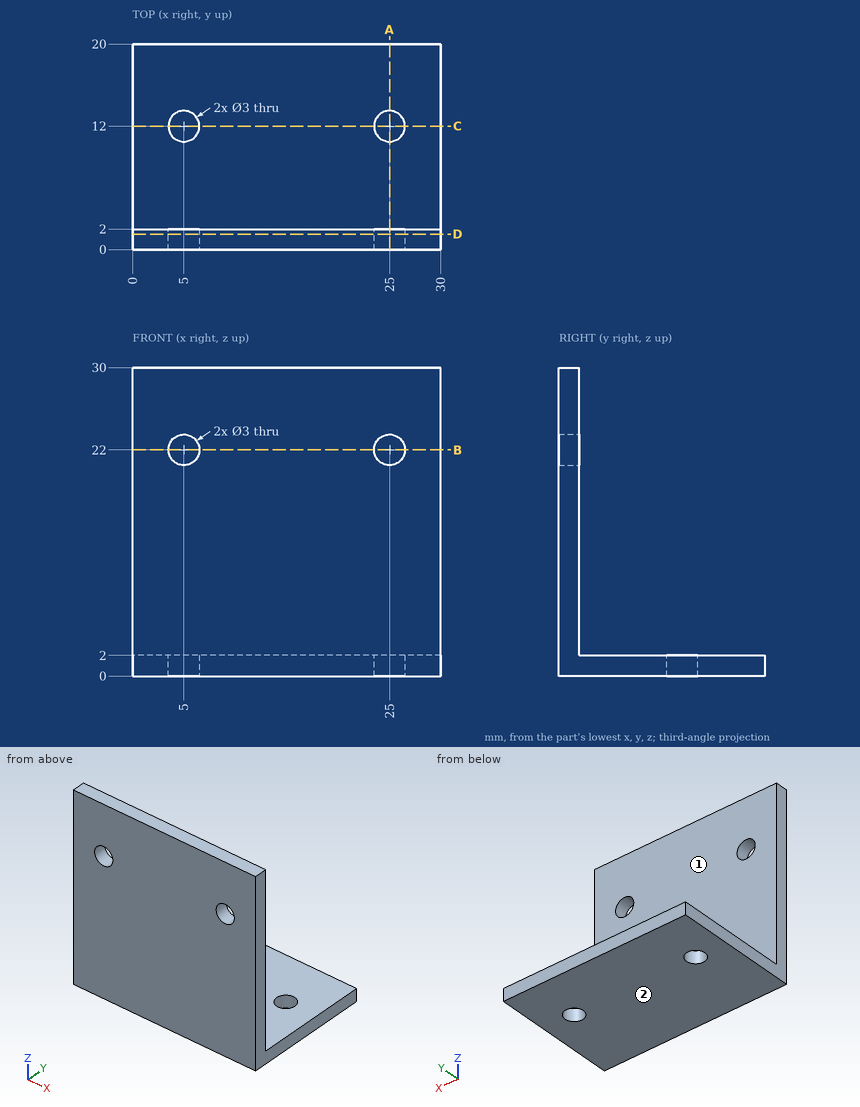
Answer from the drawing. Dimensions are ordinates in mm from the lowest x, y and z of the part. A direction names the side the tool comes from. Give positions to 0.01 mm unless a question says otherwise; leave off trailing zeros. Write each loop counter-clockwise with the first axis right and the second up, starting at its lowest first coordinate (ties: lowest second). Pieces come first, ordered by that corner, then holes. Notation, with made-up numbers: (40.5, -12) - (64.5, -12) arc R24 cw to (64.5, 14) - close; hole circle Ø6 at (63.5, 7). An arc over 180 degrees is marked (long way). Answer in a Markdown table with one row per item. Add a question column.
Item 1: Section A-A, the plane x = 25 is taken. Write down the section's boundary in (y, z).
Item 2: Find the intervals of material crossed by L1, parallel to X at y = 1.15, z = 22; L2, parallel to Y at x = 5, z = 0.65; L3, parallel to Z at x = 5, y = 1.1, in increasing order.
Item 3: Flat-ended cylindrical pins translate along their axes: P1, Ø1.5, axis at x = 24.5, z = 25, coming from the +Y side; P2, Ø4, axis at x = 21.5, y = 12, coming from the +Z side. Find the tip coordinate at first contact, or state that the pin passes through.
Item 4: A tool of negligible diameter and unlimited length cuts with its end or side. For the marked faces 1 and 2, from which of +Z, -Z, +X, -X, +Y, -Y can it reach the whole face along a straight path? Write none if from no direction.
Item 5: Section B-B, the plane z = 22 is taken. Write down the section's boundary in (x, y), and give its area (3 significant figures).
Item 6: Section D-D, the plane y = 1.5 is taken. Write down the section's boundary in (x, z), and give its area (3 significant figures).
Recorded:
| question | item | result |
|---|---|---|
| 1 | outline | (0, 0) - (10.5, 0) - (10.5, 2) - (2, 2) - (2, 20.5) - (0, 20.5) - close; (0, 23.5) - (2, 23.5) - (2, 30) - (0, 30) - close; (13.5, 0) - (20, 0) - (20, 2) - (13.5, 2) - close |
| 2 | L1 | x = 0 to 3.5, 6.5 to 23.5, 26.5 to 30 |
| 2 | L2 | y = 0 to 10.5, 13.5 to 20 |
| 2 | L3 | z = 0 to 20.5, 23.5 to 30 |
| 3 | P1 | stops at y = 2 |
| 3 | P2 | stops at z = 2 |
| 4 | face 1 | +Z, +X, -X, +Y |
| 4 | face 2 | -Z, +X, -X, +Y, -Y |
| 5 | outline | (0, 0) - (3.5, 0) - (3.5, 2) - (0, 2) - close; (6.5, 0) - (23.5, 0) - (23.5, 2) - (6.5, 2) - close; (26.5, 0) - (30, 0) - (30, 2) - (26.5, 2) - close |
| 5 | area | 48.0 mm2 |
| 6 | outline | (0, 0) - (30, 0) - (30, 30) - (0, 30) - close; hole circle Ø3 at (5, 22); hole circle Ø3 at (25, 22) |
| 6 | area | 886 mm2 |
